```python
from build123d import *

# Parameters (mm, degrees)
SKETCH_1_W      = 50
SKETCH_1_H      = 160
EXTRUDE_1_DEPTH = 10
SKETCH_2_R      = 6
EXTRUDE_2_DEPTH = 300
SKETCH_3_W      = 50
SKETCH_3_H      = 160
EXTRUDE_3_DEPTH = 10


with BuildPart() as part:
    # 草图1 → 凸台-拉伸1 (new body)
    with BuildSketch(Plane(origin=(0, 0, 0), x_dir=(1, 0, 0), z_dir=(0, 1, 0))):
        with Locations((-25, 80)):
            Rectangle(SKETCH_1_W, SKETCH_1_H)
    extrude(amount=EXTRUDE_1_DEPTH)

    # 草图2 → 凸台-拉伸2 (add)
    with BuildSketch(Plane(origin=(0, 10, 0), x_dir=(1, 0, 0), z_dir=(0, 1, 0))):
        with Locations(Location((-25, 120, 0), (0, 0, 270))):
            Circle(SKETCH_2_R)
        with Locations(Location((-25, 80, 0), (0, 0, 270))):
            Circle(SKETCH_2_R)
        with Locations(Location((-25, 40, 0), (0, 0, 270))):
            Circle(SKETCH_2_R)
    extrude(amount=EXTRUDE_2_DEPTH)

    # 草图3 → 凸台-拉伸3 (add)
    with BuildSketch(Plane(origin=(0, 310, 0), x_dir=(1, 0, 0), z_dir=(0, 1, 0))):
        with Locations((-25, 80)):
            Rectangle(SKETCH_3_W, SKETCH_3_H)
    extrude(amount=EXTRUDE_3_DEPTH)


solid = part.part
```
The model under review builds one solid part; all positions refer to its coordinate system, in mm. A direction names the side the tool comes from. Give positions to 0.01 mm unless a question says otherwise; leave off trailing zeros. Write each loop counter-clockwise with the first axis right and the second up, starting at its lowest first coordinate (ties: lowest second). Pieces come first, ordered by that corner, then holes. Notation, with made-up numbers: M 12.25,64 L 55.25,64 A15 ccw 55.25,92 Z; hole C 34,35 d7. An arc over 180 degrees is marked long. Answer in a Markdown table with one row per item.
Item 1: Tool access review of faces 1 (the face through (-25, 158, -86)), 2 (the face through (-25, 5, -160)): name each direction out of +Z, -Z, +X, -X, +Y, -Y from which nothing blocks a thin tool from reaching the whole face with its end or side.
Check sheet entries:
| item | result |
|---|---|
| face 1 | none |
| face 2 | -Z, +X, -X, +Y, -Y |
Item 2: Add section C-C on x = -46.5. Give the boundary of the cut face in (y, z).
Check sheet entries:
| item | result |
|---|---|
| outline | M 0,-160 L 10,-160 L 10,0 L 0,0 Z; M 310,-160 L 320,-160 L 320,0 L 310,0 Z |
Item 3: Add section D-D on z = -80. Give the boundary of the cut face in (x, y), plus the area to 3 significant figures.
Check sheet entries:
| item | result |
|---|---|
| outline | M -50,0 L 0,0 L 0,10 L -19,10 L -19,310 L 0,310 L 0,320 L -50,320 L -50,310 L -31,310 L -31,10 L -50,10 Z |
| area | 4,600 mm2 |
Item 4: Draft analysis for pull direction Z (two halves, no side actions). For faces 3 (the face through (-25, 315, -160)), 4 (the face through (-25, 158, -46)), 5 (the face through (-25, 158, -126)), 6 (the face through (0, 5, -79)), state which applies: +Z half, -Z half, draft (parallel to the pull), parting line (faces both ways), or undercut.
Check sheet entries:
| item | result |
|---|---|
| face 3 | -Z half |
| face 4 | undercut |
| face 5 | undercut |
| face 6 | draft |
Item 5: For line 1 along Y through (x, z) = (-33, -115.5); line 2 along X through (y, z) = (29.5, -115.5), list the stretches that pass through material, from the lowest coordinate up.
Check sheet entries:
| item | result |
|---|---|
| line 1 | 0 to 10, 310 to 320 |
| line 2 | -28.97 to -21.03 |
Item 6: Add section B-B on x = -25. Give the boundary of the cut face in (y, z), plus the area to 3 significant figures.
Check sheet entries:
| item | result |
|---|---|
| outline | M 0,-160 L 10,-160 L 10,-126 L 310,-126 L 310,-160 L 320,-160 L 320,0 L 310,0 L 310,-34 L 10,-34 L 10,0 L 0,0 Z; hole M 10,-114 L 310,-114 L 310,-86 L 10,-86 Z; hole M 10,-74 L 310,-74 L 310,-46 L 10,-46 Z |
| area | 14,000 mm2 |
Item 7: Add section A-A on z = -24.5. Give the boundary of the cut face in (x, y), plus the area to 3 significant figures.
Check sheet entries:
| item | result |
|---|---|
| outline | M -50,0 L 0,0 L 0,10 L -50,10 Z; M -50,310 L 0,310 L 0,320 L -50,320 Z |
| area | 1,000 mm2 |
Item 8: For P1, Ø8, axis at y = 80.5, z = -111.5, coming from the -X side; P2, Ø1.5, axis at x = -23, y = 256.5, coming from the -Z side; P3, Ø8, axis at x = -23.5, y = 148, coming from the -Z side, all flat-tipped, find the tip position at first contact; note any pin that passes through.
Check sheet entries:
| item | result |
|---|---|
| P1 | x = -28.97 |
| P2 | z = -125.87 |
| P3 | z = -126 |
